from build123d import *

# Parameters (mm, degrees)
SKETCH1_R           = 2.5
SKETCH1_R_2         = 1.5
BOSS_EXTRUDE1_DEPTH = 50
SKETCH2_W           = 6
SKETCH2_H           = 1.5
BOSS_EXTRUDE2_DEPTH = 5
SKETCH3_R           = 1
CUT_EXTRUDE1_DEPTH  = 4.25
FILLET1_R           = 2


with BuildPart() as part:
    # Sketch1 → Boss-Extrude1 (new body)
    with BuildSketch(Plane(origin=(0, 0, 0), x_dir=(1, 0, 0), z_dir=(0, 1, 0))):
        Circle(SKETCH1_R)
        Circle(SKETCH1_R_2, mode=Mode.SUBTRACT)
    extrude(amount=BOSS_EXTRUDE1_DEPTH)

    # Sketch2 → Boss-Extrude2 (add)
    with BuildSketch(Plane(origin=(0, 50, 0), x_dir=(1, 0, 0), z_dir=(0, 1, 0))):
        Rectangle(SKETCH2_W, SKETCH2_H)
    extrude(amount=BOSS_EXTRUDE2_DEPTH)

    # Sketch3 → Cut-Extrude1 (cut, through all)
    with BuildSketch(Plane(origin=(0, 0, -0.75), x_dir=(-1, 0, 0), z_dir=(0, 0, -1))):
        with Locations((0, 53)):
            Circle(SKETCH3_R)
    extrude(amount=-CUT_EXTRUDE1_DEPTH, mode=Mode.SUBTRACT)

    # Fillet1
    fillet1_edges = [part.edges().sort_by_distance(p)[0] for p in [
        (3, 55, 0),
        (-3, 55, 0),
    ]]
    fillet(fillet1_edges, radius=FILLET1_R)


solid = part.part
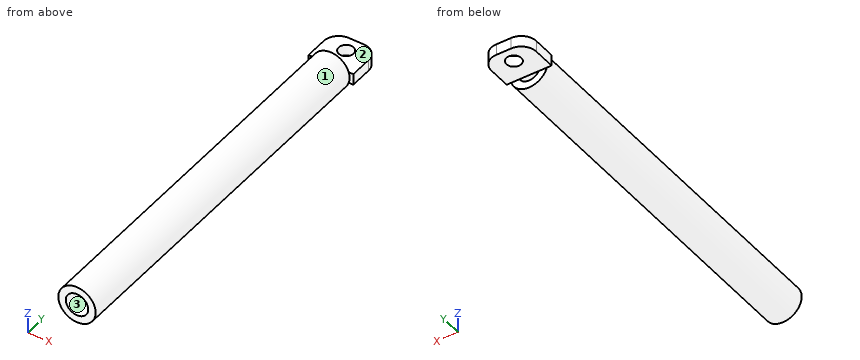
CAD build for the part. Positions are in the model's coordinates, mm. Face numbers are marked on the shaded views. Give positions to 0.01 mm unless a question says otherwise; leave off trailing zeros. Loops run counter-clockwise (first coordinate to the right, second up) from the corner with the lowest first, then second, coordinate; pieces in that order, holes last. Notation, with made-up numbers: M -26.5,-40 L 3.5,-40 A36 ccw 3.5,-6 Z; hole C -34.75,14 d4. An arc over 180 degrees is marked long. One line per question, with ' | ' between items. Start each with the question number.
1. Saw through at A-A on x = 0. Give the cut face in (y, z).
2. Flat gauge pins, fed straight in: pin 1 (1.5 mm diameter, centred on x = -0.5, y = 52, fed in from -Z); pin 2 (0.5 mm diameter, centred on x = 0.5, z = 0, fed in from -Y); pin 3 (1.5 mm diameter, centred on x = 1.5, y = 8.5, fed in from -Z). Where does each tip first touch, or does it go through?
3. Saw through at C-C on y = 35.5. Give the cut face in (x, z).
4. Saw through at D-D on z = -2. Give the cut face in (x, y), plus the area to 3 significant figures.
5. Two-plate mould, pull along Z, no slides. Class the marked faces 1, 2 and 3: pulls with the +Z half, pulls with the -Z half, needs draft (parallel to the pull), parting line crosses it, or undercut.
6. Probe L1, parallel to X at y = 14, z = -0.05; L2, parallel to Y at x = 0, z = -0.25. List the from-to ranges inside material, lowest first. Write a range as from..to.
7. Saw through at B-B on z = 0. Give the cut face in (x, y).
Result sheet:
1) outline: M 0,-2.5 L 50,-2.5 L 50,-1.5 L 0,-1.5 Z; M 0,1.5 L 50,1.5 L 50,2.5 L 0,2.5 Z; M 50,-0.75 L 52,-0.75 L 52,0.75 L 50,0.75 Z; M 54,-0.75 L 55,-0.75 L 55,0.75 L 54,0.75 Z
2) pin 1: stops at z = -0.75 | pin 2: stops at y = 50 | pin 3: stops at z = -2.38
3) outline: C 0,0 d5; hole C 0,0 d3
4) outline: M -1.5,0 L 1.5,0 L 1.5,50 L -1.5,50 Z | area: 150 mm^2
5) face 1: parting line crosses it | face 2: pulls with the +Z half | face 3: undercut
6) L1: x = -2.5..-1.5, 1.5..2.5 | L2: y = 50..52, 54..55
7) outline: M -3,50 L -2.5,50 L -2.5,0 L -1.5,0 L -1.5,50 L 1.5,50 L 1.5,0 L 2.5,0 L 2.5,50 L 3,50 L 3,53 A2 ccw 1,55 L -1,55 A2 ccw -3,53 Z; hole C 0,53 d2
